```python
from build123d import *

# Parameters (mm, degrees)
F1_DEPTH = 40.2336
F0_R     = 10.16
F2_DEPTH = 15.7734
F3_R     = 3.302


with BuildPart() as f1:
    # F0 (on Top) → F1 (new body)
    with BuildSketch(Plane.XY):
        with BuildLine():
            ThreePointArc((5.042647, -28.126541), (21.916025, -18.336262), (28.575, 0))
            ThreePointArc((28.575, 0), (21.916025, 18.336262), (5.042647, 28.126541))
            ThreePointArc((5.042647, 28.126541), (-28.575, 0), (5.042647, -28.126541))
        make_face()
        with BuildLine():
            ThreePointArc((13.447765, -4.826), (-14.2875, 0), (13.447765, 4.826))
            Line((13.447765, 4.826), (16.4084, 4.826))
            Line((16.4084, 4.826), (16.4084, -4.826))
            Line((16.4084, -4.826), (13.447765, -4.826))
        make_face(mode=Mode.SUBTRACT)
    extrude(amount=F1_DEPTH)

    # F0 (on Top) → F2 (join)
    with BuildSketch(Plane.XY):
        with BuildLine():
            ThreePointArc((5.042647, -28.126541), (21.916025, -18.336262), (28.575, 0))
            ThreePointArc((28.575, 0), (21.916025, 18.336262), (5.042647, 28.126541))
            ThreePointArc((5.042647, 28.126541), (-28.575, 0), (5.042647, -28.126541))
        make_face()
        with BuildLine():
            ThreePointArc((13.447765, -4.826), (-14.2875, 0), (13.447765, 4.826))
            Line((13.447765, 4.826), (16.4084, 4.826))
            Line((16.4084, 4.826), (16.4084, -4.826))
            Line((16.4084, -4.826), (13.447765, -4.826))
        make_face(mode=Mode.SUBTRACT)
        with BuildLine():
            ThreePointArc((5.042647, 28.126541), (21.916025, 18.336262), (28.575, 0))
            ThreePointArc((28.575, 0), (21.916025, -18.336262), (5.042647, -28.126541))
            Line((5.042647, -28.126541), (57.336765, -18.751028))
            ThreePointArc((57.336765, -18.751028), (73.025, 0), (57.336765, 18.751028))
            Line((57.336765, 18.751028), (5.042647, 28.126541))
        make_face()
        with Locations((53.975, 0)):
            Circle(F0_R, mode=Mode.SUBTRACT)
    extrude(amount=F2_DEPTH)

    # F3
    f3_edges = [f1.edges().sort_by_distance(p)[0] for p in [
        (-5.042647, 28.126541, 40.2336),
    ]]
    fillet(f3_edges, radius=F3_R)


solid = f1.part
```
Build history of the part. All positions in model axes, mm. A direction names the side the tool comes from. Round coordinates to 2 decimals unless told otherwise and drop trailing zeros. Write each loop counter-clockwise with the first axis right and the second up, starting at its lowest first coordinate (ties: lowest second). Pieces come first, ordered by that corner, then holes.
1) 3-axis set-ups, long thin cutter, end or side, ignore diameter. For faces 1 (the flat face through (30.824, -23.504, 7.776)), 2 (the flat face through (15, -4.826, 20)): which of +Z, -Z, +X, -X, +Y, -Y reach the whole face in a straight line?
2) Drill centre lines: probe 1 along Y at (x, z) = (0, 30) (1 decimal); probe 2 along X at (y, z) = (-1, 3); probe 3 along X at (y, z) = (-6.5, 6.5). Where is each one in solid material? Low to high.
3) Pin check, flat tips, straight feed: pin 1 (3.5 mm diameter, centred on x = 14.5, z = 15, fed in from +Y); pin 2 (3 mm diameter, centred on x = -14, z = 33, fed in from -Y); pin 3 (10 mm diameter, centred on x = -10.5, z = 5, fed in from +Y); pin 4 (4 mm diameter, centred on x = 13.5, y = 1, fed in from +Z). Stop position of each tip, or through.
4) Band-saw the part on B-B, the plane z = 6.5. Give the number of separate pieces and of enclosed holes in the cut face, and give its area (3 significant figures).
5) Band-saw the part on D-D, the plane x = 31. List the corners of the cut face in (y, z), and give its area (3 significant figures).
6) Mould opens along X. For faces 3 (the flat face through (39, 0, 15.773)), 4 (the flat face through (16.408, 0, 20)), 5 (the cylindrical face through (73.02, -0.37, 7.78)) say: +X half, -X half, draft (parallel to the pull), parting line (faces both ways), or undercut.
Ans:
1. face 1: +Z, -Z, +X, -Y
1. face 2: +Z, -Z
2. probe 1: y = -28.6 to -14.3, 14.3 to 28.6
2. probe 2: x = -28.56 to -14.25, 16.41 to 43.86, 64.09 to 73
2. probe 3: x = -27.83 to -12.72, 12.72 to 46.17, 61.78 to 71.88
3. pin 1: stops at y = 26.74
3. pin 2: stops at y = -25.7
3. pin 3: stops at y = 28.04
3. pin 4: passes through
4. separate pieces: 1
4. enclosed holes: 2
4. area: 3,470 mm2
5. outline: (-23.47, 0) - (23.47, 0) - (23.47, 15.77) - (-23.47, 15.77) - close
5. area: 740 mm2
6. face 3: draft
6. face 4: undercut
6. face 5: +X half
